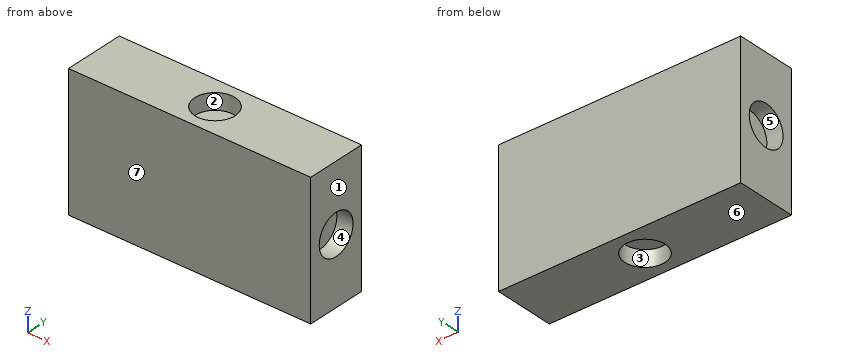
from build123d import *

# Parameters (mm, degrees)
SKETCH1_W           = 76.2
SKETCH1_H           = 41.91
BOSS_EXTRUDE1_DEPTH = 19.05
SKETCH5_R           = 6.35
CUT_EXTRUDE1_DEPTH  = 5.08
SKETCH2_R           = 6.35
CUT_EXTRUDE2_DEPTH  = 5.08
CUT_EXTRUDE3_START  = -5.08
SKETCH3_R           = 6.35
CUT_EXTRUDE3_DEPTH  = 5.08
CUT_EXTRUDE4_START  = -5.08
SKETCH4_R           = 6.35
CUT_EXTRUDE4_DEPTH  = 5.08


with BuildPart() as part:
    # Sketch1 → Boss-Extrude1 (new body)
    with BuildSketch(Plane(origin=(0, 0, 0), x_dir=(1, 0, 0), z_dir=(0, 1, 0))):
        Rectangle(SKETCH1_W, SKETCH1_H)
    extrude(amount=BOSS_EXTRUDE1_DEPTH)

    # Sketch5 → Cut-Extrude1 (cut)
    with BuildSketch(Plane(origin=(38.1, 0, 0), x_dir=(0, 0, -1), z_dir=(1, 0, 0))):
        with Locations((0, 9.525)):
            Circle(SKETCH5_R)
    extrude(amount=-CUT_EXTRUDE1_DEPTH, mode=Mode.SUBTRACT)

    # Sketch2 → Cut-Extrude2 (cut)
    with BuildSketch(Plane.XY.offset(20.955)):
        with Locations((0, 9.525)):
            Circle(SKETCH2_R)
    extrude(amount=-CUT_EXTRUDE2_DEPTH, mode=Mode.SUBTRACT)

    # Sketch3 → Cut-Extrude3 (cut)
    with BuildSketch(Plane(origin=(0, 0, -20.955), x_dir=(-1, 0, 0), z_dir=(0, 0, -1)).offset(CUT_EXTRUDE3_START)):
        with Locations(Location((0, 9.525, 0), (0, 0, 180))):
            Circle(SKETCH3_R)
    extrude(amount=CUT_EXTRUDE3_DEPTH, mode=Mode.SUBTRACT)

    # Sketch4 → Cut-Extrude4 (cut)
    with BuildSketch(Plane.ZY.offset(38.1).offset(CUT_EXTRUDE4_START)):
        with Locations(Location((0, 9.525, 0), (0, 0, 180))):
            Circle(SKETCH4_R)
    extrude(amount=CUT_EXTRUDE4_DEPTH, mode=Mode.SUBTRACT)


solid = part.part
Part model, mm, in its own coordinate system. Face numbers are marked on the shaded views. A direction names the side the tool comes from. Round coordinates to 2 decimals unless told otherwise and drop trailing zeros. Write each loop counter-clockwise with the first axis right and the second up, starting at its lowest first coordinate (ties: lowest second). Pieces come first, ordered by that corner, then holes. Notation, with made-up numbers: (71.5, 46) - (88.5, 46) arc R23 ccw to (88.5, 59) - close; hole circle Ø2 at (68, 82.5). An arc over 180 degrees is marked (long way). Use CSV: the item, a comma, the result in double quotes.
Item 1: Wall check: L1, parallel to Y at x = 0, z = 18.3 (3 decimals); L2, parallel to X at y = 6.25, z = -18.5; L3, parallel to X at y = 4.5, z = -17.5. Give the ranges that are in metal, low to high.
Results list:
L1,"y = 0 to 3.175, 15.875 to 19.05"
L2,"x = -38.1 to -5.44, 5.44 to 38.1"
L3,"x = -38.1 to -3.88, 3.88 to 38.1"
Item 2: Slice it at C-C, the plane y = 14. Write the cut outline in (x, z) (3 decimals), then the cut area to 3 significant figures.
Results list:
outline,"(-38.1, -20.955) - (-4.505, -20.955) - (-4.505, -15.875) - (4.505, -15.875) - (4.505, -20.955) - (38.1, -20.955) - (38.1, -4.505) - (33.02, -4.505) - (33.02, 4.505) - (38.1, 4.505) - (38.1, 20.955) - (4.505, 20.955) - (4.505, 15.875) - (-4.505, 15.875) - (-4.505, 20.955) - (-38.1, 20.955) - (-38.1, 4.505) - (-33.02, 4.505) - (-33.02, -4.505) - (-38.1, -4.505) - close"
area,"3,010 mm²"
Item 3: Slice it at A-A, the plane z = 0. Write the cut outline in (x, y) (3 decimals).
Results list:
outline,"(-38.1, 0) - (38.1, 0) - (38.1, 3.175) - (33.02, 3.175) - (33.02, 15.875) - (38.1, 15.875) - (38.1, 19.05) - (-38.1, 19.05) - (-38.1, 15.875) - (-33.02, 15.875) - (-33.02, 3.175) - (-38.1, 3.175) - close"
Item 4: Flat gauge pins, fed straight in: P1, Ø10, axis at x = 17.5, z = 1, coming from the -Y side; P2, Ø6.5, axis at y = 9, z = 0, coming from the +X side; P3, Ø10, axis at x = 0, y = 9.525, coming from the +Z side (3 decimals). Where does each tip first touch, or does it go through?
Results list:
P1,"stops at y = 0"
P2,"stops at x = 33.02"
P3,"stops at z = 15.875"
Item 5: Tool access for the marked faces 1, 2 and 3: list every direction of +Z, -Z, +X, -X, +Y, -Y with a clear straight run to the whole face (end or side of a thin tool).
Results list:
face 1,"+Z, -Z, +X, +Y, -Y"
face 2,"+Z"
face 3,"-Z"
Item 6: Pull direction Z, two halves, no side cores. Call the marked faces 4, 5, 6 and 7: pulls with the +Z half, pulls with the -Z half, needs draft (parallel to the pull), parting line crosses it, or undercut.
Results list:
face 4,"undercut"
face 5,"undercut"
face 6,"pulls with the -Z half"
face 7,"needs draft"
Item 7: Slice it at B-B, the plane x = 0. Write the cut outline in (y, z) (3 decimals).
Results list:
outline,"(0, -20.955) - (3.175, -20.955) - (3.175, -15.875) - (15.875, -15.875) - (15.875, -20.955) - (19.05, -20.955) - (19.05, 20.955) - (15.875, 20.955) - (15.875, 15.875) - (3.175, 15.875) - (3.175, 20.955) - (0, 20.955) - close"
Item 8: Slice it at D-D, the plane z = 18. Write the cut outline in (x, y) (3 decimals), then the cut area to 3 significant figures.
Results list:
outline,"(-38.1, 0) - (38.1, 0) - (38.1, 19.05) - (-38.1, 19.05) - close; hole circle Ø12.7 at (0, 9.525)"
area,"1,320 mm²"
